```python
from build123d import *

# Parameters (mm, degrees)
F0_W     = 25
F0_H     = 25
F1_DEPTH = 16
F2_T     = -3
F4_DEPTH = 25


with BuildPart() as f1:
    # F0 (on Top) → F1 (new body)
    with BuildSketch(Plane.XY):
        with Locations((12.5, 12.5)):
            Rectangle(F0_W, F0_H)
    extrude(amount=F1_DEPTH)

    # F2
    f2_openings = [f1.faces().sort_by_distance(p)[0] for p in [
        (12.5, 12.5, 0),
    ]]
    offset(amount=F2_T, openings=f2_openings)

    # F3 (on face) → F4 (cut)
    with BuildSketch(Plane.XY.offset(16)):
        with BuildLine():
            Line((12.5, 12.5), (17.0961940777, 17.0961940777))
            ThreePointArc((17.0961940777, 17.0961940777), (12.5, 19), (7.9038059223, 17.0961940777))
            Line((7.9038059223, 17.0961940777), (12.5, 12.5))
        make_face()
        with BuildLine():
            ThreePointArc((19, 12.5), (18.5052169613, 14.9874423104), (17.0961940777, 17.0961940777))
            Line((17.0961940777, 17.0961940777), (12.5, 12.5))
            Line((12.5, 12.5), (17.0961940777, 7.9038059223))
            ThreePointArc((17.0961940777, 7.9038059223), (18.5052169613, 10.0125576896), (19, 12.5))
        make_face()
        with BuildLine():
            Line((17.0961940777, 7.9038059223), (12.5, 12.5))
            Line((12.5, 12.5), (7.9038059223, 7.9038059223))
            ThreePointArc((7.9038059223, 7.9038059223), (12.5, 6), (17.0961940777, 7.9038059223))
        make_face()
        with BuildLine():
            Line((7.9038059223, 7.9038059223), (12.5, 12.5))
            Line((12.5, 12.5), (7.9038059223, 17.0961940777))
            ThreePointArc((7.9038059223, 17.0961940777), (6, 12.5), (7.9038059223, 7.9038059223))
        make_face()
    extrude(amount=-F4_DEPTH, mode=Mode.SUBTRACT)


solid = f1.part
```
Build history of the part. All positions in model axes, mm. A direction names the side the tool comes from. Coordinates: 2 decimals unless noted, no trailing zeros. Order: outer loops, then holes, each group sorted by start corner. A loop starts at its lowest first (then second) coordinate and runs counter-clockwise, first axis right, second up.
Item 1: Saw through at D-D on y = 20. List the corners of the cut face in (x, z).
Filled in:
outline: (0, 0) - (3, 0) - (3, 13) - (22, 13) - (22, 0) - (25, 0) - (25, 16) - (0, 16) - close
Item 2: Mould opens along X. For faces 1 (the flat face through (12, 25, 8)), 2 (the flat face through (0, 12, 8)), 3 (the flat face through (3, 12, 6)) say: released by +X, released by -X, zero draft, split by the parting line, or undercut.
Filled in:
face 1: zero draft
face 2: released by -X
face 3: undercut
Item 3: Drill centre lines: L1, parallel to Y at x = 10, z = 4; L2, parallel to Y at x = 15.75, z = 13.25. Where is each one in solid material? Low to high.
Filled in:
L1: y = 0 to 3, 22 to 25
L2: y = 0 to 6.87, 18.13 to 25
Item 4: Saw through at B-B on y = 12. List the corners of the cut face in (x, z), then the cut area to 3 significant figures.
Filled in:
outline: (0, 0) - (3, 0) - (3, 13) - (6.02, 13) - (6.02, 16) - (0, 16) - close; (18.98, 13) - (22, 13) - (22, 0) - (25, 0) - (25, 16) - (18.98, 16) - close
area: 114 mm2
Item 5: Saw through at A-A on z = 14.25. List the corners of the cut face in (x, y).
Filled in:
outline: (0, 0) - (25, 0) - (25, 25) - (0, 25) - close; hole circle Ø13 at (12.5, 12.5)
Item 6: Tool access for faces 4 (the flat face through (22, 12, 6)), 5 (the flat face through (12, 0, 8)): list every direction of +Z, -Z, +X, -X, +Y, -Y with a clear straight run to the whole face (end or side of a thin tool).
Filled in:
face 4: -Z
face 5: +Z, -Z, +X, -X, -Y
